from build123d import *

# Parameters (mm, degrees)
SKETCH_1_W          = 350
SKETCH_1_H          = 250
EXTRUDE_1_DEPTH     = 30
SKETCH_2_W          = 290
SKETCH_2_H          = 210
CUT_EXTRUDE_1_DEPTH = 30
SKETCH_3_R          = 3
CUT_EXTRUDE_2_DEPTH = 351
SKETCH_4_W          = 350
SKETCH_4_H          = 250
SKETCH_4_W_2        = 330
SKETCH_4_H_2        = 230
EXTRUDE_2_DEPTH     = 150
SKETCH_5_W          = 10
SKETCH_5_H          = 230
CUT_EXTRUDE_3_DEPTH = 150


with BuildPart() as part:
    # 草图1 → 凸台-拉伸1 (new body)
    with BuildSketch(Plane.XY):
        Rectangle(SKETCH_1_W, SKETCH_1_H)
    extrude(amount=EXTRUDE_1_DEPTH)

    # 草图2 → 切除-拉伸1 (cut)
    with BuildSketch(Plane.XY.offset(30)):
        Rectangle(SKETCH_2_W, SKETCH_2_H)
    extrude(amount=-CUT_EXTRUDE_1_DEPTH, mode=Mode.SUBTRACT)

    # 草图3 → 切除-拉伸2 (cut, through all)
    with BuildSketch(Plane(origin=(175, 0, 0), x_dir=(0, 0, -1), z_dir=(1, 0, 0))):
        with Locations((-20, 85)):
            Circle(SKETCH_3_R)
    cut_extrude_2 = extrude(amount=-CUT_EXTRUDE_2_DEPTH, mode=Mode.SUBTRACT)

    # 镜向1: 切除-拉伸2 across plane
    add(cut_extrude_2.mirror(Plane.ZX), mode=Mode.SUBTRACT)

    # 草图4 → 凸台-拉伸2 (add)
    with BuildSketch(Plane.XY.offset(30)):
        Rectangle(SKETCH_4_W, SKETCH_4_H)
        Rectangle(SKETCH_4_W_2, SKETCH_4_H_2, mode=Mode.SUBTRACT)
    extrude(amount=EXTRUDE_2_DEPTH)

    # 草图5 → 切除-拉伸3 (cut)
    with BuildSketch(Plane.XY.offset(180)):
        with Locations((170, 0)):
            Rectangle(SKETCH_5_W, SKETCH_5_H)
    extrude(amount=-CUT_EXTRUDE_3_DEPTH, mode=Mode.SUBTRACT)


solid = part.part
Could you check a few things on this model? Use its own coordinates, in mm. A direction names the side the tool comes from. Give positions to 0.01 mm unless a question says otherwise; leave off trailing zeros. Loops run counter-clockwise (first coordinate to the right, second up) from the corner with the lowest first, then second, coordinate; pieces in that order, holes last. Notation, with made-up numbers: M -2,26 L 20,26 A12 cw 20,37 Z; hole C 8.25,-36.75 d8. An arc over 180 degrees is marked long. Answer as a JSON object with one key per item and string values.
Q1. If we mould it in two halves opening along X, with no side actions, what happens to faces 1 (the flat face through (175, 8.7, 29.6)), 2 (the flat face through (-145, -1, 15)), 3 (the flat face through (-2, 105, 15)), 4 (the flat face through (3, -115, 104))? For each: pulls with the +X half, pulls with the -X half, needs draft (parallel to the pull), parting line crosses it, or undercut.
Values found:
{"face 1": "pulls with the +X half", "face 2": "undercut", "face 3": "undercut", "face 4": "needs draft"}
Q2. For faces 5 (the flat face through (145, -1, 15)), 6 (the flat face through (-2, -125, 89)), 7 (the flat face through (3, 115, 106)), which set-ups out of +Z, -Z, +X, -X, +Y, -Y let a thin tool reach every point of the face, with its end or its side?
Values found:
{"face 5": "+Z, -Z", "face 6": "+Z, -Z, +X, -X, -Y", "face 7": "+Z, +X"}
Q3. If I drill on probe 1 along Y at (x, z) = (-163, 20); probe 2 along Y at (x, z) = (-23, 163); probe 3 along X at (y, z) = (34.5, 23), over which ranges is the centre line in solid material (lowest first)? Write a range as [from, to].
Values found:
{"probe 1": "y = [-125, -88], [-82, 82], [88, 125]", "probe 2": "y = [-125, -115], [115, 125]", "probe 3": "x = [-175, -145], [145, 175]"}
Q4. Suppose I cut it at A-A, the plane x = 133. List the corners of the cut face in (y, z) for me, plus the area to 3 significant figures.
Values found:
{"outline": "M -125,0 L -105,0 L -105,30 L -115,30 L -115,180 L -125,180 Z; M 105,0 L 125,0 L 125,180 L 115,180 L 115,30 L 105,30 Z", "area": "4,200 mm²"}
Q5. Suppose I cut it at B-B, the plane y = -60.5. List the corners of the cut face in (x, z) for me, plus the area to 3 significant figures.
Values found:
{"outline": "M -175,0 L -145,0 L -145,30 L -165,30 L -165,180 L -175,180 Z; M 145,0 L 175,0 L 175,30 L 145,30 Z", "area": "3,300 mm²"}
Q6. Suppose I cut it at C-C, the plane z = 52.5. List the corners of the cut face in (x, y) for me.
Values found:
{"outline": "M -175,-125 L 175,-125 L 175,-115 L -165,-115 L -165,115 L 175,115 L 175,125 L -175,125 Z"}
Q7. For P1, Ø5.5, axis at y = 85, z = 20, coming from the -X side; P2, Ø10, axis at y = 69.5, z = 139, coming from the +X side, each with a flat end and sliding along its axis, tell me the tip position at first contact or that it passes through.
Values found:
{"P1": "passes through", "P2": "stops at x = -165"}
